```python
from build123d import *

# Parameters (mm, degrees)
F3_DEPTH = 6
F5_DEPTH = 6
F6_R     = 1
F7_DEPTH = 5.501


with BuildPart() as f1:
    # F0 (on Right) → F1 (revolve)
    with BuildSketch(Plane.YZ):
        Polygon((0, 27), (0, 0), (3, 0), (3, 5), (1, 5), (1, 19), (3, 19), (3, 27), align=None)
    revolve(axis=Axis((0, 0, 14.70128), (0, 0, 1)))

    # F2 (on face) → F3 (cut)
    with BuildSketch(Plane(origin=(0, 0, 0), x_dir=(1, 0, 0), z_dir=(0, 0, -1))):
        with BuildLine():
            Line((2.5, -2.987541), (3.128111, -2.987541))
            Line((3.128111, -2.987541), (3.128111, 3.060273))
            Line((3.128111, 3.060273), (2.5, 3.060273))
            Line((2.5, 3.060273), (2.5, 1.658312))
            ThreePointArc((2.5, 1.658312), (2.872281, 0.866025), (3, 0))
            ThreePointArc((3, 0), (2.872281, -0.866025), (2.5, -1.658312))
            Line((2.5, -1.658312), (2.5, -2.987541))
        make_face()
        with BuildLine():
            Line((2.5, 1.658312), (2.5, -1.658312))
            ThreePointArc((2.5, -1.658312), (2.872281, -0.866025), (3, 0))
            ThreePointArc((3, 0), (2.872281, 0.866025), (2.5, 1.658312))
        make_face()
    extrude(amount=-F3_DEPTH, mode=Mode.SUBTRACT)

    # F4 (on face) → F5 (cut)
    with BuildSketch(Plane(origin=(0, 0, 0), x_dir=(1, 0, 0), z_dir=(0, 0, -1))):
        with BuildLine():
            Line((-5.039785, -4.02743), (-2.5, -4.02743))
            Line((-2.5, -4.02743), (-2.5, -1.658312))
            ThreePointArc((-2.5, -1.658312), (-3, 0), (-2.5, 1.658312))
            Line((-2.5, 1.658312), (-2.5, 4.430752))
            Line((-2.5, 4.430752), (-5.039785, 4.430752))
            Line((-5.039785, 4.430752), (-5.039785, -4.02743))
        make_face()
        with BuildLine():
            ThreePointArc((-2.5, 1.658312), (-3, 0), (-2.5, -1.658312))
            Line((-2.5, -1.658312), (-2.5, 1.658312))
        make_face()
    extrude(amount=-F5_DEPTH, mode=Mode.SUBTRACT)

    # F6 (on face) → F7 (cut, through all)
    with BuildSketch(Plane.YZ.offset(2.5)):
        with Locations((0, 2)):
            Circle(F6_R)
    extrude(amount=-F7_DEPTH, mode=Mode.SUBTRACT)


solid = f1.part
```
CAD build for the part. Positions are in the model's coordinates, mm. A direction names the side the tool comes from. Give positions to 0.01 mm unless a question says otherwise; leave off trailing zeros. Loops run counter-clockwise (first coordinate to the right, second up) from the corner with the lowest first, then second, coordinate; pieces in that order, holes last. Notation, with made-up numbers: M 14,27 L 40,27 A20 cw 40,33 Z; hole C -18,7 d6. An arc over 180 degrees is marked long. Use one line per item in the form item = value.
Item 1: Flat gauge pins, fed straight in: pin 1 (3 mm diameter, centred on y = 0, z = 2, fed in from -X); pin 2 (2.5 mm diameter, centred on y = 0, z = 1.5, fed in from +X); pin 3 (2 mm diameter, centred on y = 0.5, z = 8, fed in from -X). Where does each tip first touch, or does it go through?
Determined:
pin_1 = -2.5
pin_2 = 2.5
pin_3 = -1
Item 2: Drill centre lines: probe 1 along Z at (x, y) = (0.15, 2.6); probe 2 along Z at (x, y) = (-1.55, 0.1); probe 3 along Z at (x, y) = (-0.7, 0). Where is each one in solid material? Low to high. Write a range as from..to.
Determined:
probe_1 = 0..5, 19..27
probe_2 = 0..1.01, 2.99..5, 19..27
probe_3 = 0..1, 3..27
Item 3: Which spindle directions (+Z, -Z, +X, -X, +Y, -Y) get a long thin tool onto all of the face, cutting with end or side? Do faces 4 (the face through (-2.5, 1, 3)), 5 (the face through (0, 3, 3)), 6 (the face through (1, 0, 12)). Say none if no direction does.
Determined:
face_4 = -Z, -X, +Y, -Y
face_5 = +Z, -Z, +Y
face_6 = none
Item 4: Slice it at B-B (z = 2). List the corners of the cut face in (x, y), plus the area to 3 significant figures.
Determined:
outline = M -2.5,-1.66 A3 ccw 2.5,-1.66 L 2.5,-1 L -2.5,-1 Z; M -2.5,1 L 2.5,1 L 2.5,1.66 A3 ccw -2.5,1.66 Z
area = 16.0 mm2
Item 5: Two-plate mould, pull along Z, no slides. Class faces 1 (the face through (-1.15, -0.04, 5)), 2 (the face through (2.5, 1, 3)), 3 (the face through (0, 0, 27)): pulls with the +Z half, pulls with the -Z half, needs draft (parallel to the pull), parting line crosses it, or undercut.
Determined:
face_1 = undercut
face_2 = needs draft
face_3 = pulls with the +Z half
Item 6: Slice it at A-A (y = 0.4). List the corners of the cut face in (x, z), plus the area to 3 significant figures.
Determined:
outline = M -2.97,19 L -0.92,19 L -0.92,5 L -2.5,5 L -2.5,2.92 L 2.5,2.92 L 2.5,5 L 0.92,5 L 0.92,19 L 2.97,19 L 2.97,27 L -2.97,27 Z; M -2.5,0 L 2.5,0 L 2.5,1.08 L -2.5,1.08 Z
area = 89.1 mm2
Item 7: Slice it at D-D (x = 0.6). List the corners of the cut face in (y, z).
Determined:
outline = M -2.94,0 L 2.94,0 L 2.94,5 L 0.8,5 L 0.8,19 L 2.94,19 L 2.94,27 L -2.94,27 L -2.94,19 L -0.8,19 L -0.8,5 L -2.94,5 Z; hole C 0,2 d2
Item 8: Slice it at C-C (x = 1.6). List the corners of the cut face in (y, z), plus the area to 3 significant figures.
Determined:
outline = M -2.54,0 L 2.54,0 L 2.54,5 L -2.54,5 Z; M -2.54,19 L 2.54,19 L 2.54,27 L -2.54,27 Z; hole C 0,2 d2
area = 62.8 mm2
